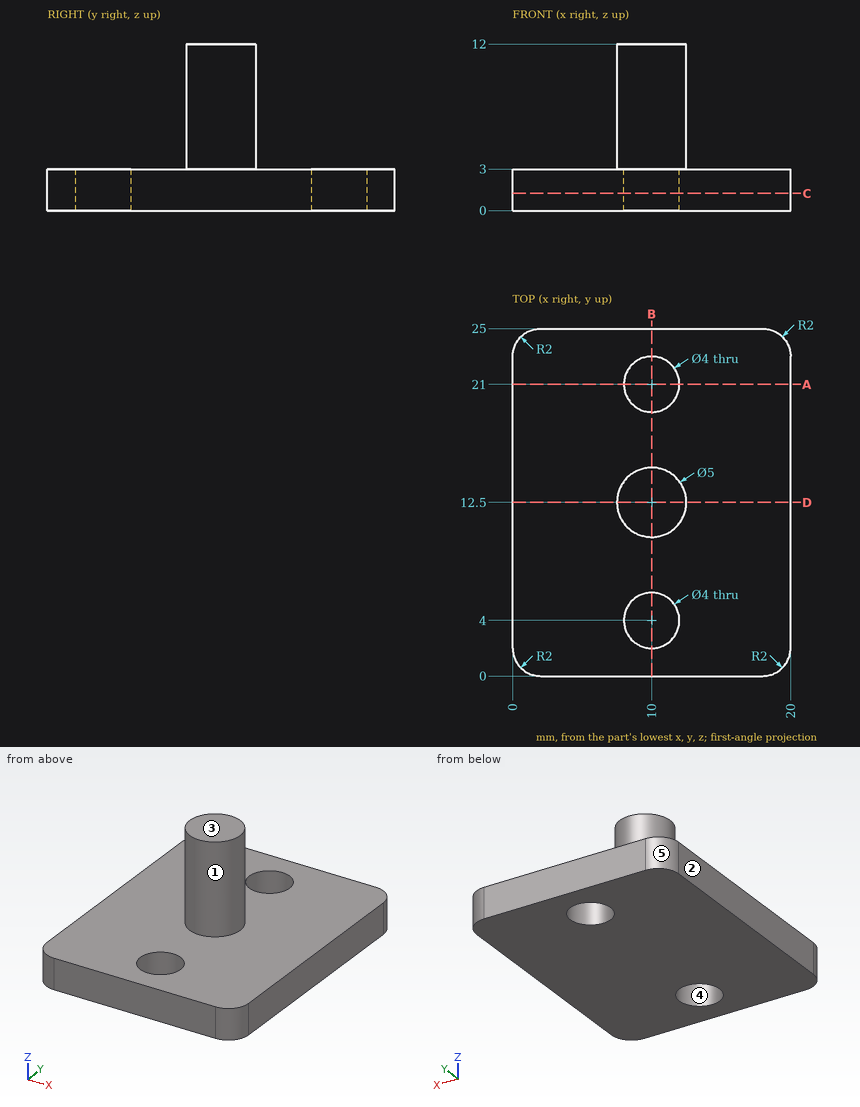
Could you check a few things on this drawing? It's one solid part, dimensions in mm from its lowest x, y, z. A direction names the side the tool comes from. Round coordinates to 2 decimals unless told otherwise and drop trailing zeros. Loops run counter-clockwise (first coordinate to the right, second up) from the corner with the lowest first, then second, coordinate; pieces in that order, holes last. Notation, with made-up numbers: M 87.5,48.25 L 146.5,48.25 A15 cw 146.5,64.25 Z; hole C -8,8 d8. An arc over 180 degrees is marked long. Write each question's results on one line, items separated by ' | '. Start each with the question number.
(1) I want a section at B-B (x = 10). Please give me the cut outline in (y, z).
(2) I want a section at C-C (z = 1.25). Please give me the cut outline in (x, y).
(3) Thinking about a two-plate mould opening in X: for the marked faces 3, 4 and 5, which applies, pulls with the +X half, pulls with the -X half, needs draft (parallel to the pull), parting line crosses it, or undercut?
(4) Will these pins go through, and if not, where does the flat tip stop? P1, Ø1, axis at y = 19.5, z = 4, coming from the +X side; P2, Ø6.5, axis at x = 10, y = 21, coming from the +Z side; P3, Ø3, axis at y = 12, z = 9.5, coming from the +X side.
(5) I want a section at D-D (y = 12.5). Please give me the cut outline in (x, z), then the cut area to 3 significant figures.
(6) On a 3-axis mill with a long thin cutter (end or side, diameter ignored), from which of +Z, -Z, +X, -X, +Y, -Y can I reach the whole of each face in a straight line? I mean the marked faces 1 and 2. Say none if no direction works.
(7) I want a section at A-A (y = 21). Please give me the cut outline in (x, z), then the cut area to 3 significant figures.
(8) If I drill on probe 1 along Y at (x, z) = (10, 1.8); probe 2 along X at (y, z) = (4, 2.2); probe 3 along Z at (x, y) = (11.75, 7.5), over which ranges is the centre line in solid material (lowest first)? Write a range as from..to.
Solved:
1) outline: M 0,0 L 2,0 L 2,3 L 0,3 Z; M 6,0 L 19,0 L 19,3 L 15,3 L 15,12 L 10,12 L 10,3 L 6,3 Z; M 23,0 L 25,0 L 25,3 L 23,3 Z
2) outline: M 0,2 A2 ccw 2,0 L 18,0 A2 ccw 20,2 L 20,23 A2 ccw 18,25 L 2,25 A2 ccw 0,23 Z; hole C 10,4 d4; hole C 10,21 d4
3) face 3: needs draft | face 4: undercut | face 5: pulls with the -X half
4) P1: passes through | P2: stops at z = 3 | P3: stops at x = 12.5
5) outline: M 0,0 L 20,0 L 20,3 L 12.5,3 L 12.5,12 L 7.5,12 L 7.5,3 L 0,3 Z | area: 105 mm²
6) face 1: +Z | face 2: +Z, -Z, -X, +Y, -Y
7) outline: M 0,0 L 8,0 L 8,3 L 0,3 Z; M 12,0 L 20,0 L 20,3 L 12,3 Z | area: 48.0 mm²
8) probe 1: y = 0..2, 6..19, 23..25 | probe 2: x = 0..8, 12..20 | probe 3: z = 0..3
